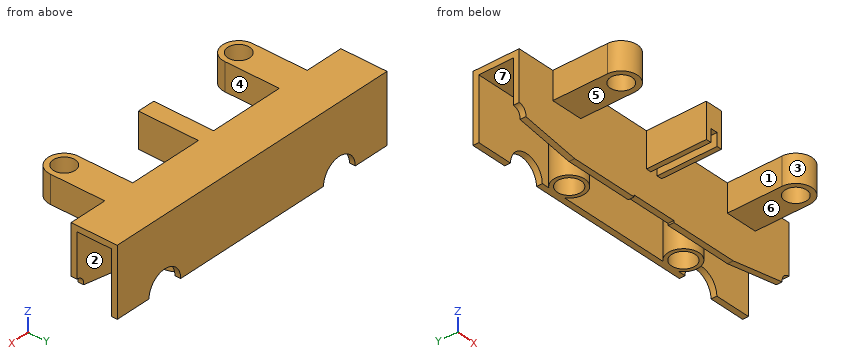
from build123d import *

# Parameters (mm, degrees)
F1_DEPTH       = 85
F3_DEPTH       = 3.2
F4_W           = 25
F4_H           = 1
F5_DEPTH       = 3.2
F6_R           = 6.5
F7_DEPTH       = 34
F9_DEPTH       = 33
F11_R          = 6
F12_DEPTH      = 5
F12_DEPTH_BACK = 10.2
F13_DEPTH      = 9.4


with BuildPart() as f1:
    # F0 (on Right) → F1 (new body, symmetric)
    with BuildSketch(Plane.YZ):
        Polygon((2.7508442084, 0), (2.7508442084, 37.2), (-22.6491557916, 37.2), (-22.6491557916, 0), (-19.4491557916, 0), (-19.4491557916, 34), (-0.4491557916, 34), (-0.4491557916, 0), align=None)
    extrude(amount=F1_DEPTH, both=True)

    # F2 (on face) → F3 (cut, through all)
    with BuildSketch(Plane(origin=(0, 2.7508442084, 0), x_dir=(-1, 0, 0), z_dir=(0, 1, 0))):
        with BuildLine():
            Line((-65, 0), (-45, 0))
            ThreePointArc((-45, 0), (-55, 10), (-65, 0))
        make_face()
        with BuildLine():
            ThreePointArc((65, 0), (55, 10), (45, 0))
            Line((45, 0), (65, 0))
        make_face()
    extrude(amount=-F3_DEPTH, mode=Mode.SUBTRACT)

    # F4 (on face) → F5 (cut, through all)
    with BuildSketch(Plane.XZ.offset(22.6491557916)):
        Polygon((-80.8183589196, 5.2831472434), (-85, 6), (-85, 0), (-50, 0), align=None)
        Polygon((80.8183589196, 5.2831472434), (50, 0), (85, 0), (85, 6), align=None)
        with Locations((0, 0.5)):
            Rectangle(F4_W, F4_H)
        with BuildLine():
            Line((-85, 10.2426406871), (-85, 6))
            Line((-85, 6), (-80.8183589196, 5.2831472434))
            ThreePointArc((-80.8183589196, 5.2831472434), (-81.7564411003, 8.7348355826), (-85, 10.2426406871))
        make_face()
        with BuildLine():
            Line((85, 6), (85, 10.2426406871))
            ThreePointArc((85, 10.2426406871), (81.7564411003, 8.7348355826), (80.8183589196, 5.2831472434))
            Line((80.8183589196, 5.2831472434), (85, 6))
        make_face()
    extrude(amount=-F5_DEPTH, mode=Mode.SUBTRACT)

    # F6 (on face) → F7 (join, through all)
    with BuildSketch(Plane(origin=(0, 0, 34), x_dir=(1, 0, 0), z_dir=(0, 0, -1))):
        with BuildLine():
            ThreePointArc((40.8905171703, 0.4491557916), (36, 15.9013383128), (31.1094828297, 0.4491557916))
            Line((31.1094828297, 0.4491557916), (40.8905171703, 0.4491557916))
        make_face()
        with Locations((36, 7.4013383128)):
            Circle(F6_R, mode=Mode.SUBTRACT)
        with BuildLine():
            Line((-40.8905171703, 0.4491557916), (-31.1094828297, 0.4491557916))
            ThreePointArc((-31.1094828297, 0.4491557916), (-36, 15.9013383128), (-40.8905171703, 0.4491557916))
        make_face()
        with Locations((-36, 7.4013383128)):
            Circle(F6_R, mode=Mode.SUBTRACT)
    extrude(amount=F7_DEPTH)

    # F8 (on face) → F9 (join)
    with BuildSketch(Plane.XZ.offset(22.6491557916)):
        Polygon((-2, 18), (-2, 25), (2, 25), (2, 18), (4.8, 18), (4.8, 27.8), (-4.8, 27.8), (-4.8, 18), align=None)
    extrude(amount=F9_DEPTH)

    # F11 (on offset) → F12 (join, two sides)
    with BuildSketch(Plane(origin=(0, 0, 27), x_dir=(1, 0, 0), z_dir=(0, 0, -1))) as f12_sk:
        with BuildLine():
            Line((-46.2, 22.6491557916), (-46.2, 52.6491557916))
            ThreePointArc((-46.2, 52.6491557916), (-55, 43.8491557916), (-63.8, 52.6491557916))
            Line((-63.8, 52.6491557916), (-63.8, 22.6491557916))
            Line((-63.8, 22.6491557916), (-46.2, 22.6491557916))
        make_face()
        with BuildLine():
            ThreePointArc((-63.8, 52.6491557916), (-55, 43.8491557916), (-46.2, 52.6491557916))
            ThreePointArc((-46.2, 52.6491557916), (-55, 61.4491557916), (-63.8, 52.6491557916))
        make_face()
        with Locations((-55, 52.6491557916)):
            Circle(F11_R, mode=Mode.SUBTRACT)
        with BuildLine():
            Line((63.8, 22.6491557916), (63.8, 52.6491557916))
            ThreePointArc((63.8, 52.6491557916), (55, 43.8491557916), (46.2, 52.6491557916))
            Line((46.2, 52.6491557916), (46.2, 22.6491557916))
            Line((46.2, 22.6491557916), (63.8, 22.6491557916))
        make_face()
        with BuildLine():
            ThreePointArc((46.2, 52.6491557916), (55, 43.8491557916), (63.8, 52.6491557916))
            ThreePointArc((63.8, 52.6491557916), (55, 61.4491557916), (46.2, 52.6491557916))
        make_face()
        with Locations((55, 52.6491557916)):
            Circle(F11_R, mode=Mode.SUBTRACT)
    extrude(amount=F12_DEPTH)
    extrude(f12_sk.sketch, amount=-F12_DEPTH_BACK)

    # F13 (add, through all): a face of the model
    f13_faces = [f1.faces().sort_by_distance(p)[0] for p in [
        (0, -39.1491557916, 27.8),
    ]]
    extrude(f13_faces, amount=F13_DEPTH)


solid = f1.part
Design review of the part built by this model. Coordinates are the model's own, in mm. Face numbers are marked on the shaded views. A direction names the side the tool comes from. Coordinates: 2 decimals unless noted, no trailing zeros. Loops run counter-clockwise (first coordinate to the right, second up) from the corner with the lowest first, then second, coordinate; pieces in that order, holes last.
Item 1: For the marked faces 4, 5, 6 and 7, list the 3-axis set-ups (+Z, -Z, +X, -X, +Y, -Y) from which the entire face can be reached by the end or side of a thin tool; tool diameter is ignored.
Completed:
face 4: +Z, -Z, -Y
face 5: -Z, -X, -Y
face 6: -Z, +X, -Y
face 7: -Z
Item 2: Wall thickness on L1, parallel to X at y = -37.5, z = 33; L2, parallel to Y at x = 36, z = 13; L3, parallel to Y at x = 55, z = 29.25: over which ranges is each line inside the solid? List them lowest first.
Completed:
L1: x = -63.8 to -46.2, -4.8 to 4.8, 46.2 to 63.8
L2: y = -22.65 to -19.45, -15.9 to -13.9, -0.9 to 2.75
L3: y = -61.45 to -58.65, -46.65 to -19.45, -0.45 to 2.75
Item 3: Add section C-C (x = -55). Write out the cut boundary in (y, z).
Completed:
outline: (-61.45, 22) - (-58.65, 22) - (-58.65, 37.2) - (-61.45, 37.2) - close; (-46.65, 22) - (-22.65, 22) - (-22.65, 0.86) - (-19.45, 0.86) - (-19.45, 34) - (-0.45, 34) - (-0.45, 10) - (2.75, 10) - (2.75, 37.2) - (-46.65, 37.2) - close
Item 4: Add section A-A (y = -33). Write out the cut boundary in (x, z), and give its area (3 significant figures).
Completed:
outline: (-63.8, 22) - (-46.2, 22) - (-46.2, 37.2) - (-63.8, 37.2) - close; (-4.8, 18) - (-2, 18) - (-2, 25) - (2, 25) - (2, 18) - (4.8, 18) - (4.8, 37.2) - (-4.8, 37.2) - close; (46.2, 22) - (63.8, 22) - (63.8, 37.2) - (46.2, 37.2) - close
area: 691 mm2
Item 5: Clearance check with flat-ended pins moving along their axes: pin 1 (3 mm diameter, centred on x = -3, y = -43, fed in from -Z); pin 2 (4 mm diameter, centred on x = -36.5, y = -4.5, fed in from -Z); pin 3 (8 mm diameter, centred on y = -15.5, z = 6, fed in from -X); pin 4 (11 mm diameter, centred on x = -55, y = -52.65, fed in from -Z). State where each tip first meets the part, or that it passes through.
Completed:
pin 1: stops at z = 18
pin 2: stops at z = 34
pin 3: stops at x = -80.81
pin 4: passes through
Item 6: Add section B-B (z = 32.5). Write out the cut boundary in (x, y).
Completed:
outline: (-85, -22.65) - (-63.8, -22.65) - (-63.8, -52.65) arc R8.8 ccw to (-46.2, -52.65) - (-46.2, -22.65) - (-4.8, -22.65) - (-4.8, -55.65) - (4.8, -55.65) - (4.8, -22.65) - (46.2, -22.65) - (46.2, -52.65) arc R8.8 ccw to (63.8, -52.65) - (63.8, -22.65) - (85, -22.65) - (85, -19.45) - (-85, -19.45) - close; (-85, -0.45) - (-40.89, -0.45) arc R8.5 ccw (long way) to (-31.11, -0.45) - (31.11, -0.45) arc R8.5 ccw (long way) to (40.89, -0.45) - (85, -0.45) - (85, 2.75) - (-85, 2.75) - close; hole circle Ø12 at (-55, -52.65); hole circle Ø13 at (-36, -7.4); hole circle Ø13 at (36, -7.4); hole circle Ø12 at (55, -52.65)
Item 7: Add section D-D (y = -51). Write out the cut boundary in (x, z), and give its area (3 significant figures).
Completed:
outline: (-63.8, 22) - (-60.77, 22) - (-60.77, 37.2) - (-63.8, 37.2) - close; (-49.23, 22) - (-46.2, 22) - (-46.2, 37.2) - (-49.23, 37.2) - close; (-4.8, 18) - (-2, 18) - (-2, 25) - (2, 25) - (2, 18) - (4.8, 18) - (4.8, 37.2) - (-4.8, 37.2) - close; (46.2, 22) - (49.23, 22) - (49.23, 37.2) - (46.2, 37.2) - close; (60.77, 22) - (63.8, 22) - (63.8, 37.2) - (60.77, 37.2) - close
area: 341 mm2
Item 8: Draft analysis for pull direction X (two halves, no side actions). For the marked faces 1, 2 and 3, state which applies: pulls with the +X half, pulls with the -X half, needs draft (parallel to the pull), parting line crosses it, or undercut.
Completed:
face 1: undercut
face 2: needs draft
face 3: undercut
